```python
from build123d import *

# Parameters (mm, degrees)
ESQUISSE1_R        = 73.8
ESQUISSE1_R_2      = 62
BOSS_EXTRU_1_DEPTH = 30
ESQUISSE2_W        = 2
ESQUISSE2_H        = 15
ESQUISSE2_W_2      = 30
ESQUISSE2_H_2      = 2
BOSS_EXTRU_2_DEPTH = 20


with BuildPart() as part:
    # Esquisse1 → Boss.-Extru.1 (new body)
    with BuildSketch(Plane(origin=(0, 0, 0), x_dir=(1, 0, 0), z_dir=(0, 1, 0))):
        with Locations(Location((0, 0, 0), (0, 0, 270))):
            Circle(ESQUISSE1_R)
        with Locations(Location((0, 0, 0), (0, 0, 270))):
            Circle(ESQUISSE1_R_2, mode=Mode.SUBTRACT)
    extrude(amount=BOSS_EXTRU_1_DEPTH)

    # Esquisse2 → Boss.-Extru.2 (add)
    with BuildSketch(Plane(origin=(0, 30, 0), x_dir=(1, 0, 0), z_dir=(0, 1, 0))):
        with Locations((-69.786402014, 7.5)):
            Rectangle(ESQUISSE2_W, ESQUISSE2_H)
        with Locations((-69.786402014, -7.5)):
            Rectangle(ESQUISSE2_W, ESQUISSE2_H)
        with Locations((-63.786402014, -7.5)):
            Rectangle(ESQUISSE2_W, ESQUISSE2_H)
        with Locations((-63.786402014, 7.5)):
            Rectangle(ESQUISSE2_W, ESQUISSE2_H)
        with Locations((0, 69.786402014)):
            Rectangle(ESQUISSE2_W_2, ESQUISSE2_H_2)
        with Locations((0, 63.786402014)):
            Rectangle(ESQUISSE2_W_2, ESQUISSE2_H_2)
        with Locations((63.786402014, -7.5)):
            Rectangle(ESQUISSE2_W, ESQUISSE2_H)
        with Locations((63.786402014, 7.5)):
            Rectangle(ESQUISSE2_W, ESQUISSE2_H)
        with Locations((69.786402014, 7.5)):
            Rectangle(ESQUISSE2_W, ESQUISSE2_H)
        with Locations((69.786402014, -7.5)):
            Rectangle(ESQUISSE2_W, ESQUISSE2_H)
        with Locations((0, -69.786402014)):
            Rectangle(ESQUISSE2_W_2, ESQUISSE2_H_2)
        with Locations((0, -63.786402014)):
            Rectangle(ESQUISSE2_W_2, ESQUISSE2_H_2)
    extrude(amount=BOSS_EXTRU_2_DEPTH)


solid = part.part
```
Design review of the part built by this model. Coordinates are the model's own, in mm. A direction names the side the tool comes from. Give positions to 0.01 mm unless a question says otherwise; leave off trailing zeros. Order: outer loops, then holes, each group sorted by start corner. A loop starts at its lowest first (then second) coordinate and runs counter-clockwise, first axis right, second up. Notation, with made-up numbers: (35.5, -9) -> (68.5, -9) arc R18 ccw to (68.5, 9) -> close; hole circle Ø9 at (33.25, 18). An arc over 180 degrees is marked (long way). Write item = value, one per line. Start each with the question number.
(1) For faces 1 (the face through (0, 40, -62.786)), 2 (the face through (-70.786, 40, 0)), 3 (the face through (70.786, 40, 0)), 4 (the face through (-62.786, 40, 0)), list the 3-axis set-ups (+Z, -Z, +X, -X, +Y, -Y) from which the entire face can be reached by the end or side of a thin tool; tool diameter is ignored.
(2) We need section B-B on y = 36.5. State how many separate pieces and enclosed holes the cut face has, plus the area to 3 significant figures.
(3) For pin 1 (6 mm diameter, centred on x = 53.5, z = -40, fed in from +Y); pin 2 (8 mm diameter, centred on y = 29, z = -30, fed in from +X); pin 3 (12 mm diameter, centred on y = 24.5, z = -10.5, fed in from +X), all flat-tipped, find the tip position at first contact; note any pin that passes through.
(4) We need section A-A on z = 0. Write out the cut boundary in (x, y).
(5) We need section C-C on x = -23. Write out the cut boundary in (y, z), plus the area to 3 significant figures.
(6) To check wall thickness, follow line 1 along Z through (x, y) = (-14, 39); line 2 along X through (y, z) = (11.5, 0); line 3 along Y through (x, z) = (57, -42). State the ranges of each line that lie inside material, in increasing order.
(7) Mouldability with a two-part tool opening along Z and no side actions: class faces 5 (the face through (0, 40, 70.786)), 6 (the face through (68.786, 40, 0)), 7 (the face through (0, 40, 68.786)), 8 (the face through (22.17, 14.79, 70.39)) as +Z half, -Z half, draft (parallel to the pull), parting line (faces both ways), or undercut.
(8) We need section D-D on y = 14.5. Write out the cut boundary in (x, z), plus the area to 3 significant figures.
Numbers:
q1.face_1 = +X, -X, +Y
q1.face_2 = +Z, -Z, -X, +Y
q1.face_3 = +Z, -Z, +X, +Y
q1.face_4 = +Z, -Z, +Y
q2.separate_pieces = 8
q2.enclosed_holes = 0
q2.area = 480 mm^2
q3.pin_1 = 30
q3.pin_2 = 69.07
q3.pin_3 = 73.66
q4.outline = (-73.8, 0) -> (-62, 0) -> (-62, 30) -> (-62.79, 30) -> (-62.79, 50) -> (-64.79, 50) -> (-64.79, 30) -> (-68.79, 30) -> (-68.79, 50) -> (-70.79, 50) -> (-70.79, 30) -> (-73.8, 30) -> close; (62, 0) -> (73.8, 0) -> (73.8, 30) -> (70.79, 30) -> (70.79, 50) -> (68.79, 50) -> (68.79, 30) -> (64.79, 30) -> (64.79, 50) -> (62.79, 50) -> (62.79, 30) -> (62, 30) -> close
q5.outline = (0, -70.12) -> (30, -70.12) -> (30, -57.58) -> (0, -57.58) -> close; (0, 57.58) -> (30, 57.58) -> (30, 70.12) -> (0, 70.12) -> close
q5.area = 753 mm^2
q6.line_1 = -70.79 to -68.79, -64.79 to -62.79, 62.79 to 64.79, 68.79 to 70.79
q6.line_2 = -73.8 to -62, 62 to 73.8
q6.line_3 = 0 to 30
q7.face_5 = +Z half
q7.face_6 = draft
q7.face_7 = undercut
q7.face_8 = parting line
q8.outline = circle Ø147.6 at (0, 0); hole circle Ø124 at (0, 0)
q8.area = 5,030 mm^2
